```python
from build123d import *

# Parameters (mm, degrees)
SKETCH1_W           = 40
SKETCH1_H           = 50
BOSS_EXTRUDE1_DEPTH = 2.5
SKETCH2_W           = 40
SKETCH2_H           = 2.5
BOSS_EXTRUDE2_DEPTH = 50
FILLET1_R           = 4
FILLET2_R           = 1.5


with BuildPart() as part:
    # Sketch1 → Boss-Extrude1 (new body)
    with BuildSketch(Plane(origin=(0, 0, 0), x_dir=(1, 0, 0), z_dir=(0, 1, 0))):
        with Locations((20, 25)):
            Rectangle(SKETCH1_W, SKETCH1_H)
    extrude(amount=BOSS_EXTRUDE1_DEPTH)

    # Sketch2 → Boss-Extrude2 (add)
    with BuildSketch(Plane(origin=(0, 2.5, 0), x_dir=(1, 0, 0), z_dir=(0, 1, 0))):
        with Locations((20, 48.75)):
            Rectangle(SKETCH2_W, SKETCH2_H)
        with Locations((20, 1.25)):
            Rectangle(SKETCH2_W, SKETCH2_H)
    extrude(amount=BOSS_EXTRUDE2_DEPTH)

    # Fillet1
    fillet1_edges = [part.edges().sort_by_distance(p)[0] for p in [
        (20, 0, -50),
        (20, 0, 0),
    ]]
    fillet(fillet1_edges, radius=FILLET1_R)

    # Fillet2
    fillet2_edges = [part.edges().sort_by_distance(p)[0] for p in [
        (20, 2.5, -47.5),
        (20, 2.5, -2.5),
    ]]
    fillet(fillet2_edges, radius=FILLET2_R)


solid = part.part
```
Design review of the part built by this model. Coordinates are the model's own, in mm. A direction names the side the tool comes from. Round coordinates to 2 decimals unless told otherwise and drop trailing zeros. Order: outer loops, then holes, each group sorted by start corner. A loop starts at its lowest first (then second) coordinate and runs counter-clockwise, first axis right, second up. Notation, with made-up numbers: M -33.75,50 L -7.75,50 A25 cw -7.75,86 Z; hole C 40.5,-38 d7. An arc over 180 degrees is marked long. Put each result on its own line as item: value.
Q1. Consider section C-C (z = -27). State the section outline as (x, y) points, and give its area (3 significant figures).
Reported:
outline: M 0,0 L 40,0 L 40,2.5 L 0,2.5 Z
area: 100 mm²
Q2. Consider section A-A (y = 31). State the section outline as (x, z) points.
Reported:
outline: M 0,-50 L 40,-50 L 40,-47.5 L 0,-47.5 Z; M 0,-2.5 L 40,-2.5 L 40,0 L 0,0 Z
Q3. Draft analysis for pull direction Z (two halves, no side actions). For faces 1 (the face through (20.28, 2.93, -2.95)), 2 (the face through (20, 2.5, -25)), 3 (the face through (20, 52.5, -49)), 4 (the face through (20.28, 1.203, -1.141)), state which applies: released by +Z, released by -Z, zero draft, split by the parting line, or undercut.
Reported:
face 1: undercut
face 2: undercut
face 3: zero draft
face 4: released by +Z
Q4. Consider section B-B (x = 6). State the section outline as (y, z) points, and give its area (3 significant figures).
Reported:
outline: M 0,-46 A4 ccw 4,-50 L 52.5,-50 L 52.5,-47.5 L 4,-47.5 A1.5 cw 2.5,-46 L 2.5,-4 A1.5 cw 4,-2.5 L 52.5,-2.5 L 52.5,0 L 4,0 A4 ccw 0,-4 Z
area: 369 mm²
Q5. Machinability: for faces 5 (the face through (20.28, 1.141, -48.797)), 6 (the face through (20, 28, -47.5)), which of the approach directions +Z, -Z, +X, -X, +Y, -Y give a long, thin tool a straight path to every point of the face, cutting with its end or side? Answer none if there is none.
Reported:
face 5: -Z, +X, -X, -Y
face 6: +X, -X, +Y
Q6. Insertion check: pin 1 Ø8 at (x, z) = (7.5, -36) entering from +Y. The pin has a flat end and moves straight along its axis. Give the tip position at first contact, or say it passes through.
Reported:
pin 1: y = 2.5
Q7. To check wall thickness, follow line 1 (Z direction, x = 22.5, y = 31); line 2 (Y direction, x = 17, z = -45); line 3 (Z direction, x = 4.5, y = 3). State the ranges of each line that lie inside material, in increasing order.
Reported:
line 1: -50 to -47.5, -2.5 to 0
line 2: 0 to 2.5
line 3: -49.87 to -47.12, -2.88 to -0.13
